Geometry: see drawing. Coordinates: mm, zero at the bounding-box minimum. A direction names the side the tool comes from. Round coordinates to 2 decimals unless told otherwise and drop trailing zeros. Loops run counter-clockwise (first coordinate to the right, second up) from the corner with the lowest first, then second, coordinate; pieces in that order, holes last. Notation, with made-up numbers: (21.25, 36) - (38.25, 36) arc R19 cw to (38.25, 55) - close; hole circle Ø1 at (25.25, -2). An arc over 180 degrees is marked (long way). Use CSV: the item, a comma, the result in double quotes. Start each with the question number.
1. Cut plane C-C (y = 37). Return loops of the section in (x, z), and give its area (3 significant figures).
2. Access query for the marked faces 1, 2 and 3. Directions: +Z, -Z, +X, -X, +Y, -Y. A direction counts if a zero-diameter tool reaches every point of the face in a straight line with its end or side. Return the directions, or none.
3. Pin query (flat end, axial travel): P1, Ø2, axis at x = 7, z = 9.5, coming from the +Y side; P2, Ø2, axis at x = 7.5, y = 4, coming from the +Z side; P3, Ø10, axis at x = 13.5, y = 19, coming from the +Z side. Return the tip coordinate at first contact, or that it passes through.
4. Cut plane D-D (z = 15.5). Return loops of the section in (x, y).
5. Cut plane B-B (x = 10). Return loops of the section in (y, z), and give its area (3 significant figures).
6. Pull-direction query (Y, two-part tool) for the marked faces 4, 5, 6 and 7; classes: +Y half, -Y half, draft (parallel to the pull), parting line (faces both ways), or undercut.
7. Cut plane A-A (y = 2). Return loops of the section in (x, z).
8. Material intervals for probe 1 along X at (y, z) = (2, 27.65); probe 2 along Z at (x, y) = (18, 31.5); probe 3 along Y at (x, z) = (1.5, 30), sorted ascending. Write a range as from..to.
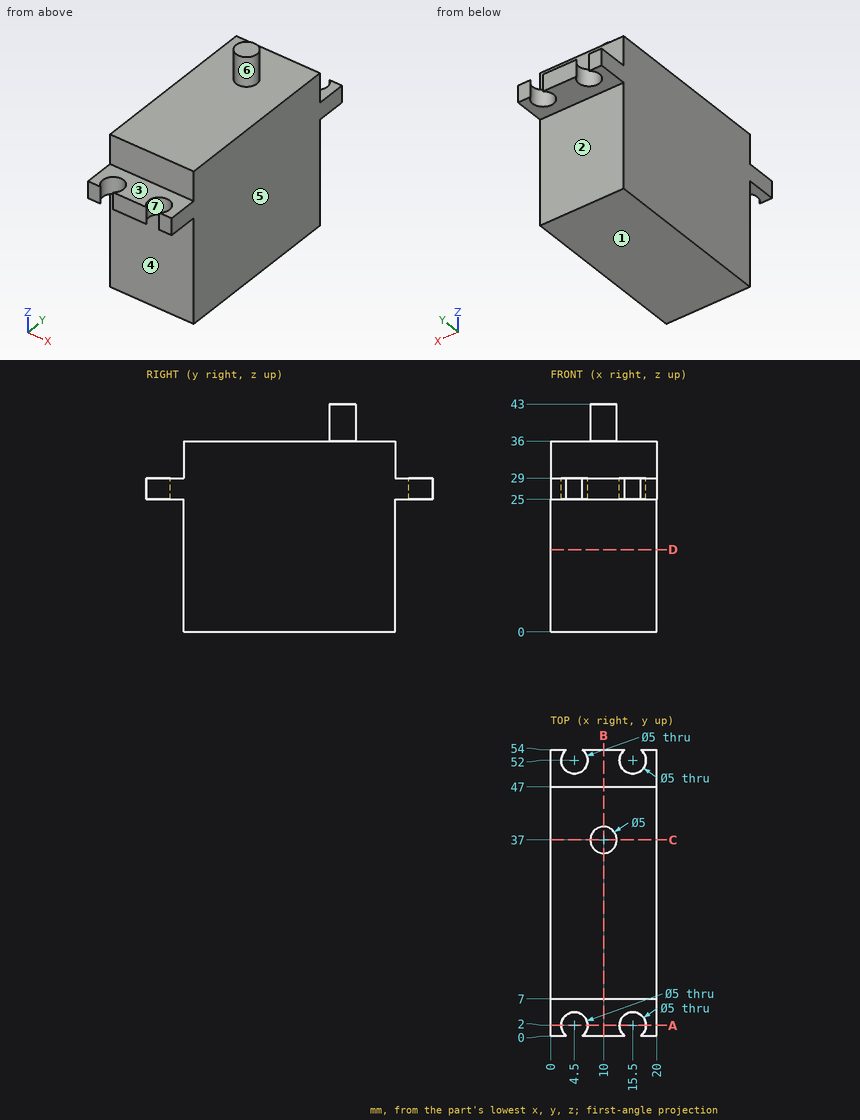
Established:
1,outline,"(0, 0) - (20, 0) - (20, 36) - (12.5, 36) - (12.5, 43) - (7.5, 43) - (7.5, 36) - (0, 36) - close"
1,area,"755 mm2"
2,face 1,"-Z, +X, -X, +Y, -Y"
2,face 2,"-Z, +X, -X, +Y"
2,face 3,"+Z, +X, -X, -Y"
3,P1,"stops at y = 47"
3,P2,"stops at z = 29"
3,P3,"stops at z = 36"
4,outline,"(0, 7) - (20, 7) - (20, 47) - (0, 47) - close"
5,outline,"(0, 25) - (7, 25) - (7, 0) - (47, 0) - (47, 25) - (54, 25) - (54, 29) - (47, 29) - (47, 36) - (39.5, 36) - (39.5, 43) - (34.5, 43) - (34.5, 36) - (7, 36) - (7, 29) - (0, 29) - close"
5,area,"1,530 mm2"
6,face 4,"-Y half"
6,face 5,"draft"
6,face 6,"parting line"
6,face 7,"undercut"
7,outline,"(0, 25) - (2, 25) - (2, 29) - (0, 29) - close; (7, 25) - (13, 25) - (13, 29) - (7, 29) - close; (18, 25) - (20, 25) - (20, 29) - (18, 29) - close"
8,probe 1,"x = 0..2, 7..13, 18..20"
8,probe 2,"z = 0..36"
8,probe 3,"y = 7..47"
